from build123d import *

# Parameters (mm, degrees)
F0_W     = 250
F0_H     = 100
F0_R     = 12
F1_DEPTH = 25


with BuildPart() as f1:
    # F0 (on Front) → F1 (new body)
    with BuildSketch(Plane.XZ):
        with Locations((125, 50)):
            Rectangle(F0_W, F0_H)
        with BuildLine():
            ThreePointArc((225, 37), (237, 25), (225, 13))
            Line((225, 13), (25, 13))
            ThreePointArc((25, 13), (13, 25), (25, 37))
            Line((25, 37), (225, 37))
        make_face(mode=Mode.SUBTRACT)
        with Locations((25, 70)):
            Circle(F0_R, mode=Mode.SUBTRACT)
        with BuildLine():
            ThreePointArc((237, 70), (225, 58), (213, 70))
            ThreePointArc((213, 70), (225, 82), (237, 70))
        make_face(mode=Mode.SUBTRACT)
    extrude(amount=F1_DEPTH)


solid = f1.part
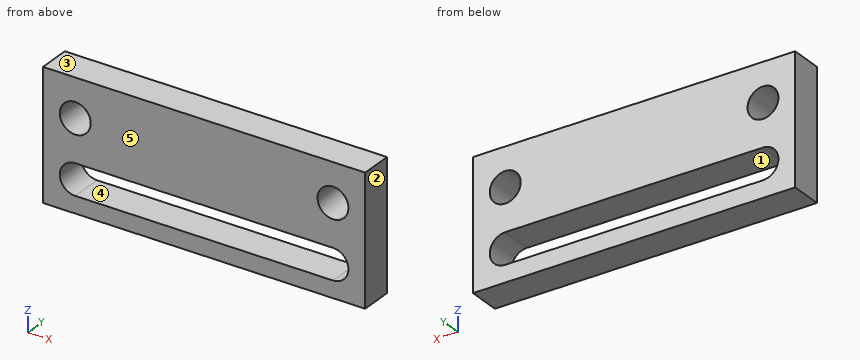
Build history of the part. All positions in model axes, mm. Face numbers are marked on the shaded views. A direction names the side the tool comes from. Coordinates: 2 decimals unless noted, no trailing zeros. Order: outer loops, then holes, each group sorted by start corner. A loop starts at its lowest first (then second) coordinate and runs counter-clockwise, first axis right, second up. Notation, with made-up numbers: M 73,50 L 83,50 A27 ccw 83,74 Z; hole C -28.5,75 d9. An arc over 180 degrees is marked long. One line per question, with ' | ' between items. Start each with the question number.
Q1. Saw through at A-A (z = 25). List the corners of the cut face in (x, y), then the cut area to 3 significant figures.
Q2. Saw through at D-D (z = 70). List the corners of the cut face in (x, y), then the cut area to 3 significant figures.
Q3. Flat gauge pins, fed straight in: pin 1 Ø14.5 at (x, z) = (25, 70) entering from -Y; pin 2 Ø8 at (x, z) = (119.5, 79.5) entering from +Y. Where does each tip first touch, or does it go through?
Q4. Probe L1, parallel to Z at x = 25, y = -13.5; L2, parallel to Z at x = 67, y = -22; L3, parallel to X at y = -20.25, z = 66. List the from-to ranges inside material, lowest first. Write a range as from..to.
Q5. Two-plate mould, pull along Z, no slides. Class the marked faces 1, 2 and 3: +Z half, -Z half, draft (parallel to the pull), parting line (faces both ways), or undercut.
Q6. 3-axis set-ups, long thin cutter, end or side, ignore diameter. For the marked faces 4 and 5: which of +Z, -Z, +X, -X, +Y, -Y reach the whole face in a straight line?
Q7. Saw through at B-B (x = 183.5). List the corners of the cut face in (y, z), then the cut area to 3 significant figures.
Q8. Saw through at C-C (y = -20.5). List the corners of the cut face in (x, z), then the cut area to 3 significant figures.
Check values:
1) outline: M 0,-25 L 13,-25 L 13,0 L 0,0 Z; M 237,-25 L 250,-25 L 250,0 L 237,0 Z | area: 650 mm2
2) outline: M 0,-25 L 13,-25 L 13,0 L 0,0 Z; M 37,-25 L 213,-25 L 213,0 L 37,0 Z; M 237,-25 L 250,-25 L 250,0 L 237,0 Z | area: 5,050 mm2
3) pin 1: passes through | pin 2: stops at y = 0
4) L1: z = 0..13, 37..58, 82..100 | L2: z = 0..13, 37..100 | L3: x = 0..13.69, 36.31..213.69, 236.31..250
5) face 1: undercut | face 2: draft | face 3: +Z half
6) face 4: +Y, -Y | face 5: +Z, -Z, +X, -X, -Y
7) outline: M -25,0 L 0,0 L 0,13 L -25,13 Z; M -25,37 L 0,37 L 0,100 L -25,100 Z | area: 1,900 mm2
8) outline: M 0,0 L 250,0 L 250,100 L 0,100 Z; hole C 25,70 d24; hole M 25,13 L 225,13 A12 ccw 225,37 L 25,37 A12 ccw Z; hole C 225,70 d24 | area: 18,800 mm2
